Verification items for the finished model (mm, model axes). A direction names the side the tool comes from. Round coordinates to 2 decimals unless told otherwise and drop trailing zeros. Loops run counter-clockwise (first coordinate to the right, second up) from the corner with the lowest first, then second, coordinate; pieces in that order, holes last. Notation, with made-up numbers: M -15,-16.75 L -7,-16.75 A20 ccw -7,6.25 Z; hole C 70,-10 d7. An arc over 180 degrees is marked long. Answer as CSV lines item,"result".
```python
from build123d import *

# Parameters (mm, degrees)
ESQUISSE3_W             = 80
ESQUISSE3_H             = 80
BOSS_EXTRU_1_DEPTH      = 2
BOSS_EXTRU_2_DEPTH      = 49
ESQUISSE7_R             = 2.05
ENL_V_MAT_EXTRU_1_DEPTH = 30
ESQUISSE8_W             = 7.1
ESQUISSE8_H             = 3.4
ENL_V_MAT_EXTRU_2_DEPTH = 9
ESQUISSE9_W             = 7.1
ESQUISSE9_H             = 3.4
ENL_V_MAT_EXTRU_3_DEPTH = 9
ESQUISSE10_W            = 2
ESQUISSE10_H            = 2
ENL_V_MAT_EXTRU_4_DEPTH = 74


with BuildPart() as part:
    # Esquisse3 → Boss.-Extru.1 (new body)
    with BuildSketch(Plane.XY):
        with Locations((40, 40)):
            Rectangle(ESQUISSE3_W, ESQUISSE3_H)
    extrude(amount=BOSS_EXTRU_1_DEPTH)

    # Esquisse6 → Boss.-Extru.2 (add)
    with BuildSketch(Plane.XY.offset(2)):
        Polygon((0, 0), (80, 0), (80, 80), (0, 80), (0, 77), (1.5, 78.5), (3, 77), (3, 70), (13, 70), (13, 77), (70, 77), (70, 70), (77, 70), (77, 10), (70, 10), (70, 3), (13, 3), (13, 10), (3, 10), (3, 3), (1.5, 1.5), (0, 3), align=None)
    extrude(amount=BOSS_EXTRU_2_DEPTH)

    # Esquisse7 → Enlèv. mat.-Extru.1 (cut)
    with BuildSketch(Plane.XY.offset(51)):
        with Locations((8, 75)):
            Circle(ESQUISSE7_R)
        with Locations((8, 5)):
            Circle(ESQUISSE7_R)
        with Locations((75, 5)):
            Circle(ESQUISSE7_R)
        with Locations((75, 75)):
            Circle(ESQUISSE7_R)
    extrude(amount=-ENL_V_MAT_EXTRU_1_DEPTH, mode=Mode.SUBTRACT)

    # Esquisse8 → Enlèv. mat.-Extru.2 (cut)
    with BuildSketch(Plane.XZ):
        with Locations((8, 46.3)):
            Rectangle(ESQUISSE8_W, ESQUISSE8_H)
        with Locations((75, 46.3)):
            Rectangle(ESQUISSE8_W, ESQUISSE8_H)
    extrude(amount=-ENL_V_MAT_EXTRU_2_DEPTH, mode=Mode.SUBTRACT)

    # Esquisse9 → Enlèv. mat.-Extru.3 (cut)
    with BuildSketch(Plane(origin=(0, 80, 0), x_dir=(1, 0, 0), z_dir=(0, 1, 0))):
        with Locations((75, -46.3)):
            Rectangle(ESQUISSE9_W, ESQUISSE9_H)
        with Locations((8, -46.3)):
            Rectangle(ESQUISSE9_W, ESQUISSE9_H)
    extrude(amount=-ENL_V_MAT_EXTRU_3_DEPTH, mode=Mode.SUBTRACT)

    # Esquisse10 → Enlèv. mat.-Extru.4 (cut)
    with BuildSketch(Plane.ZY.offset(-3)):
        with Locations((38, 71)):
            Rectangle(ESQUISSE10_W, ESQUISSE10_H)
        with Locations((38, 9)):
            Rectangle(ESQUISSE10_W, ESQUISSE10_H)
    extrude(amount=-ENL_V_MAT_EXTRU_4_DEPTH, mode=Mode.SUBTRACT)


solid = part.part
```
1) Section check C-C (y = 49). Record the cut outline in (x, z).
Here are the results:
outline,"M 0,0 L 80,0 L 80,51 L 77,51 L 77,2 L 0,2 Z"
2) Section check B-B (x = 75). State how many separate pieces and enclosed holes the cut face has, plus the area to 3 significant figures.
Here are the results:
separate pieces,"3"
enclosed holes,"0"
area,"853 mm^2"
3) Go/stop test with flat-tipped pins: pin 1 (5 mm diameter, centred on x = 68.5, z = 18, fed in from -Y); pin 2 (5.5 mm diameter, centred on y = 8, z = 30, fed in from -X); pin 3 (8 mm diameter, centred on y = 22, z = 34.5, fed in from -X); pin 4 (2 mm diameter, centred on x = 61.5, y = 23, fed in from +Z). Record where each tip stops, or that it passes through.
Here are the results:
pin 1,"stops at y = 0"
pin 2,"stops at x = 3"
pin 3,"stops at x = 77"
pin 4,"stops at z = 2"
4) Material ranges on probe 1 along Y at (x, z) = (8, 29.5); probe 2 along X at (y, z) = (73.5, 45); probe 3 along Y at (x, z) = (21, 16), recorded low to high.
Here are the results:
probe 1,"y = 0 to 2.95, 7.05 to 10, 70 to 72.95, 77.05 to 80"
probe 2,"x = 3 to 4.45, 11.55 to 13, 70 to 71.45, 78.55 to 80"
probe 3,"y = 0 to 3, 77 to 80"
5) Section check D-D (z = 11.5). Record the cut outline in (x, y), plus the area to 4 significant figures.
Here are the results:
outline,"M 0,0 L 80,0 L 80,80 L 0,80 L 0,77 L 1.5,78.5 L 3,77 L 3,70 L 13,70 L 13,77 L 70,77 L 70,70 L 77,70 L 77,10 L 70,10 L 70,3 L 13,3 L 13,10 L 3,10 L 3,3 L 1.5,1.5 L 0,3 Z"
area,"935.5 mm^2"
6) Set-up check for faces 4 (the flat face through (4.45, 4, 46)), 5 (the cylindrical face through (72.95, 5.09, 32.97)), 6 (the flat face through (73, 71, 37)), 7 (the flat face through (6, 77, 44.6)), 8 (the flat face through (3, 7, 26)): record each of +Z, -Z, +X, -X, +Y, -Y from which the full face is reachable in a straight line by a thin tool's end or side.
Here are the results:
face 4,"-Y"
face 5,"+Z"
face 6,"-X"
face 7,"+Y"
face 8,"+Z, -X"
7) Section check A-A (z = 29.5). Record the cut outline in (x, y).
Here are the results:
outline,"M 0,0 L 80,0 L 80,80 L 0,80 L 0,77 L 1.5,78.5 L 3,77 L 3,70 L 13,70 L 13,77 L 70,77 L 70,70 L 77,70 L 77,10 L 70,10 L 70,3 L 13,3 L 13,10 L 3,10 L 3,3 L 1.5,1.5 L 0,3 Z; hole C 8,5 d4.1; hole C 8,75 d4.1; hole C 75,5 d4.1; hole C 75,75 d4.1"
8) Draft check along Y on faces 1 (the flat face through (8, 9, 46)), 2 (the flat face through (13, 73, 26)), 3 (the flat face through (4.45, 76, 46)). Enter one of: +Y half, -Y half, draft (parallel to the pull), parting line (faces both ways), or undercut.
Here are the results:
face 1,"-Y half"
face 2,"undercut"
face 3,"draft"
